Autodesk Inventor part; units mm, degrees
ref_plane "YZ Plane" through (0, 0, 0) normal (1, 0, 0) x (0, 1, 0)
ref_plane "XZ Plane" through (0, 0, 0) normal (0, 1, 0) x (-1, 0, 0)
ref_plane "XY Plane" through (0, 0, 0) normal (0, 0, 1) x (1, 0, 0)
sketch "Base" plane through (0, 0, 0) normal (0, 0, 1) x (1, 0, 0)
  circle A0 centre (0, 0) radius 7
  circle A1 centre (0, 0) radius 17
  line L0 (-32.4, 0) -> (75.4, 0) construction
  line L1 (5.8143, 15.9748) -> (27.7249, 8)
  line L2 (27.7249, 8) -> (46.7497, 8)
  line L3 (46.7497, 8) -> (53, 16)
  line L4 (53, 16) -> (60, 16)
  line L5 (60, 16) -> (60, 0)
  line L6 (5.8143, -15.9748) -> (27.7249, -8)
  line L7 (27.7249, -8) -> (46.7497, -8)
  line L8 (46.7497, -8) -> (53, -16)
  line L9 (53, -16) -> (60, -16)
  line L10 (60, -16) -> (60, 0)
  point P0 (5.8143, -15.9748)
  dimension "d1" = 34
  dimension "d0" = 14
  dimension "d2" = 16
  dimension "d3" = 128
  dimension "d4" = 7
  dimension "d6" = 160
  dimension "d7" = 60
  dimension "d8" = 16
extrude "BaseFeature" add sketch "Base" along normal mid plane 5
sketch "Mount" plane through (0, 0, 2.5) normal (0, 0, 1) x (1, 0, 0)
  line L0 (60, 16) -> (53, 16)
  line L1 (60, -16) -> (60, 16)
  line L2 (53, -16) -> (60, -16)
  line L3 (46.7497, -8) -> (53, -16)
  line L4 (53, 16) -> (46.7497, 8)
  line L5 (46.7497, 8) -> (46.7497, -8)
  point P0 (0, 0)
extrude "MountFeature" add sketch "Mount" along normal blind 4
sketch "MountTransition" plane through (27.7249, -8, -2.5) normal (0, -1, 0) x (1, 0, 0)
  line L0 (0, 5) -> (19.0249, 5)
  line L1 (0, 5) -> (19.0249, 9)
  line L2 (19.0249, 5) -> (19.0249, 9)
  point P0 (-27.7249, 2.5)
extrude "MountTransitionFeature" add sketch "MountTransition" against normal up to surface (16 mm away)
sketch "HubMount" plane through (0, 0, 2.5) normal (0, 0, 1) x (1, 0, 0)
  circle A0 centre (0, -9.525) radius 1.25
  circle A1 centre (8.2489, -4.7625) radius 1.25
  circle A2 centre (8.2489, 4.7625) radius 1.25
  circle A3 centre (0, 9.525) radius 1.25
  circle A4 centre (-8.2489, 4.7625) radius 1.25
  circle A5 centre (-8.2489, -4.7625) radius 1.25
  point P0 (0, 0)
extrude "HubMountFeature" cut sketch "HubMount" against normal through all
sketch "BearingIndentation" plane through (0, 0, 2.5) normal (0, 0, 1) x (1, 0, 0)
  circle A0 centre (0, 0) radius 7
  circle A1 centre (0, 0) radius 8.05
  circle A2 centre (0, 9.525) radius 1.25
  circle A3 centre (8.2489, 4.7625) radius 1.25
  circle A4 centre (-8.2489, 4.7625) radius 1.25
  circle A5 centre (-8.2489, -4.7625) radius 1.25
  circle A6 centre (0, -9.525) radius 1.25
  circle A7 centre (8.2489, -4.7625) radius 1.25
  line L0 (-8.2489, 4.7625) -> (0, 0) construction
  line L1 (0, 9.525) -> (0, 0) construction
  line L2 (-7.6239, 5.845) -> (-6.2619, 5.0587)
  line L3 (-8.8739, 3.68) -> (-7.5119, 2.8936)
  line L4 (-1.25, 9.525) -> (-1.25, 7.9524)
  line L5 (1.25, 9.525) -> (1.25, 7.9524)
  line L6 (7.6239, 5.845) -> (6.2619, 5.0587)
  line L7 (8.8739, 3.68) -> (7.5119, 2.8936)
  line L8 (-32.4, 0) -> (75.4, 0) construction
  line L9 (-7.6239, -5.845) -> (-6.2619, -5.0587)
  line L10 (-8.8739, -3.68) -> (-7.5119, -2.8936)
  line L11 (-1.25, -9.525) -> (-1.25, -7.9524)
  line L12 (1.25, -9.525) -> (1.25, -7.9524)
  line L13 (7.6239, -5.845) -> (6.2619, -5.0587)
  line L14 (8.8739, -3.68) -> (7.5119, -2.8936)
  point P0 (1.25, -9.525)
  dimension "d47" = 16.1
extrude "BearingIndentationFeature" cut sketch "BearingIndentation" against normal blind 1 contours A1 | A1 L6 A3 L7 | L14 A7 L13 A1 | A1 L4 A2 L5 | L12 A6 L11 A1 | A1 L3 A4 L2 | L9 A5 L10 A1
sketch "Sketch16" plane through (60, -16, -2.5) normal (1, 0, 0) x (0, 0, -1)
  line L0 (0, 32) -> (-9, 32) construction
  line L1 (-9, 0) -> (-9, 32) construction
  line L2 (0, 0) -> (-9, 0) construction
  line L3 (0, 32) -> (0, 0) construction
  line L4 (-4.5, 32) -> (-4.5, 0) construction
  circle A0 centre (-4.5, 27.5) radius 2.5
  line L5 (-9, 0) -> (-9, 32)
  line L6 (-9, 16) -> (0, 16) construction
  circle A1 centre (-4.5, 4.5) radius 2.5
  point P0 (-2.5, 16)
  dimension "d65" = 5
  dimension "d66" = 4.5
  dimension "d67" = 4.5
hole "Hole2" at (60, 11.5, 2) at (60, -11.5, 2) direction (-1, 0, 0) diameter 4 depth 7 tip angle 118
equation "\"d67\" = d66"
properties part number "NeckMount"
The listing builds one solid part. Answer for the finished solid, in the listing's coordinates (mm). A direction names the side the tool comes from. Give positions to 0.01 mm unless a question says otherwise; leave off trailing zeros. Order: outer loops, then holes, each group sorted by start corner. A loop starts at its lowest first (then second) coordinate and runs counter-clockwise, first axis right, second up. Notation, with made-up numbers: (78, 6.5) -> (124, 6.5) arc R25 cw to (124, 27.5) -> close; hole circle Ø2 at (9, 37). An arc over 180 degrees is marked (long way). One line per item, written item: value.
1) Find the intervals of material crossed by line 1 (Y direction, x = 0, z = -0.5) (3 decimals); line 2 (Y direction, x = 56, z = 2); line 3 (X direction, y = -5, z = 1), in increasing order.
Reported:
line 1: y = -17 to -10.775, -8.275 to -7, 7 to 8.275, 10.775 to 17
line 2: y = -16 to -13.5, -9.5 to 9.5, 13.5 to 16
line 3: x = -16.25 to -9.48, -7.02 to -4.9, 4.9 to 7.02, 9.48 to 60
2) A tool of negligible diameter and unlimited length cuts with its end or side. For faces 1 (the flat face through (10, 0, 2.5)), 2 (the cylindrical face through (3.99, -6.99, 2.01)), 3 (the flat face through (49.83, -11.94, 1.94)), 4 (the flat face through (37, 8, 1)), 5 (the flat face through (21, 0, -2.5)), from which of +Z, -Z, +X, -X, +Y, -Y can it reach the whole face along a straight path? Write none if from no direction.
Reported:
face 1: +Z, -X, +Y, -Y
face 2: +Z
face 3: +Z, -Z, -Y
face 4: +Z, -Z, +Y
face 5: -Z, +X, -X, +Y, -Y
3) Find section C-C, the plane x = 55.5. Determine the outline of the cut face in (y, z), plus the area to 3 significant figures.
Reported:
outline: (-16, -2.5) -> (16, -2.5) -> (16, 6.5) -> (-16, 6.5) -> close; hole circle Ø4 at (-11.5, 2); hole circle Ø4 at (11.5, 2)
area: 263 mm^2
4) Determine the mould class of faces 6 (the cylindrical face through (-9.241, -5.523, 0.035)), 7 (the conical face through (52.007, 11.844, 2.045)), 8 (the cylindrical face through (-17, 0, 0)) for opening direction X: pulls with the +X half, pulls with the -X half, needs draft (parallel to the pull), parting line crosses it, or undercut.
Reported:
face 6: undercut
face 7: pulls with the +X half
face 8: parting line crosses it
5) Find section A-A, the plane x = 0. Determine the outline of the cut face in (y, z) (3 decimals).
Reported:
outline: (-17, -2.5) -> (-10.775, -2.5) -> (-10.775, 2.5) -> (-17, 2.5) -> close; (-8.275, -2.5) -> (-7, -2.5) -> (-7, 1.5) -> (-8.275, 1.5) -> close; (7, -2.5) -> (8.275, -2.5) -> (8.275, 1.5) -> (7, 1.5) -> close; (10.775, -2.5) -> (17, -2.5) -> (17, 2.5) -> (10.775, 2.5) -> close
6) Flat-ended cylindrical pins translate along their axes: P1, Ø4.5, axis at x = 32.5, z = 2, coming from the +Y side; P2, Ø2, axis at x = 56, z = 1.5, coming from the -Y side; P3, Ø9, axis at x = -3.5, y = -3.5, coming from the +Z side. Find the tip coordinate at first contact, or state that the pin passes through.
Reported:
P1: stops at y = 8
P2: stops at y = -16
P3: stops at z = 2.5
7) Find section D-D, the plane z = -1.5. Count the separate pieces of the cut face and the enclosed holes in it, plus the area to 3 significant figures.
Reported:
separate pieces: 1
enclosed holes: 7
area: 1,670 mm^2
